```python
from build123d import *

# Parameters (mm, degrees)
SKETCH1_R           = 10
BOSS_EXTRUDE3_DEPTH = 5
SKETCH3_W           = 60
SKETCH3_H           = 50
BOSS_EXTRUDE4_DEPTH = 5
SKETCH9_R           = 12.5
CUT_EXTRUDE3_DEPTH  = 2.5


with BuildPart() as part:
    # Sketch1 → Boss-Extrude3 (new body)
    with BuildSketch(Plane(origin=(0, 0, 0), x_dir=(0, 0, -1), z_dir=(1, 0, 0))):
        with BuildLine():
            Line((0, 0), (50, 0))
            Line((50, 0), (50, -20))
            Line((50, -20), (-18.826787969, -96.735647895))
            ThreePointArc((-18.826787969, -96.735647895), (-38.641397295, -98.984562701), (-43.183296189, -79.566851328))
            Line((-43.183296189, -79.566851328), (0, 0))
        make_face()
        with Locations((-29.998149885, -86.722822296)):
            Circle(SKETCH1_R, mode=Mode.SUBTRACT)
    extrude(amount=BOSS_EXTRUDE3_DEPTH)


with BuildPart() as body_2:
    # Mirror6: mirrored copy
    add(part.part.mirror(Plane(origin=(30, 0, 0), x_dir=(0, 0, 1), z_dir=(1, 0, 0))))


with BuildPart() as part_1:
    add(part.part)

    add(body_2.part)  # Boss-Extrude4 merges body 2
    # Sketch3 → Boss-Extrude4 (add)
    with BuildSketch(Plane(origin=(0, 0, 0), x_dir=(1, 0, 0), z_dir=(0, 1, 0))):
        with Locations((30, 25)):
            Rectangle(SKETCH3_W, SKETCH3_H)
    extrude(amount=BOSS_EXTRUDE4_DEPTH)

    # Sketch9 → Cut-Extrude3 (cut)
    with BuildSketch(Plane(origin=(0, 5, 0), x_dir=(1, 0, 0), z_dir=(0, 1, 0))):
        with Locations((30, 25)):
            Circle(SKETCH9_R)
    extrude(amount=-CUT_EXTRUDE3_DEPTH, mode=Mode.SUBTRACT)


solid = part_1.part
```
Verification items for the finished model (mm, model axes). A direction names the side the tool comes from. Give positions to 0.01 mm unless a question says otherwise; leave off trailing zeros. Write each loop counter-clockwise with the first axis right and the second up, starting at its lowest first coordinate (ties: lowest second). Pieces come first, ordered by that corner, then holes. Notation, with made-up numbers: M -33.75,-38 L -6.75,-38 A33 ccw -6.75,-3 Z; hole C 9.25,59 d6. An arc over 180 degrees is marked long. One line per question, with ' | ' between items.
1) Section check C-C on y = -44.5. Enter the section's corners in (x, z), plus the area to 3 significant figures.
Result:
outline: M 0,-28.03 L 5,-28.03 L 5,24.15 L 0,24.15 Z; M 55,-28.03 L 60,-28.03 L 60,24.15 L 55,24.15 Z | area: 522 mm2
2) Set-up check for faces 1 (the flat face through (0, -37, -2)), 2 (the flat face through (30, 2.5, -25)), 3 (the flat face through (57.54, -57.83, -16.07)), 4 (the flat face through (30, 0, -25)), 5 (the flat face through (30, 2, 0)): record each of +Z, -Z, +X, -X, +Y, -Y from which the full face is reachable in a straight line by a thin tool's end or side.
Result:
face 1: +Z, -Z, -X, +Y, -Y | face 2: +Y | face 3: -Z, +X, -X, -Y | face 4: +Z, -Z, -Y | face 5: +Z, +X, -X, +Y
3) Section check B-B on z = 3. Enter the section's corners in (x, y).
Result:
outline: M 0,-79.09 L 5,-79.09 L 5,-5.53 L 0,-5.53 Z; M 55,-79.09 L 60,-79.09 L 60,-5.53 L 55,-5.53 Z
4) Section check A-A on y = -84. Enter the section's corners in (x, z), plus the area to 3 significant figures.
Result:
outline: M 0,7.4 L 5,7.4 L 5,20.38 L 0,20.38 Z; M 0,39.62 L 5,39.62 L 5,44.75 L 0,44.75 Z; M 55,7.4 L 60,7.4 L 60,20.38 L 55,20.38 Z; M 55,39.62 L 60,39.62 L 60,44.75 L 55,44.75 Z | area: 181 mm2
5) Mould release check, pull along Z, two halves, no side actions. Record for faces 6 (the cylindrical face through (20.08, 3.768, -17.394)), 7 (the cylindrical face through (57.54, -99.16, 38.39)), 8 (the flat face through (57.535, -40.34, 21.894)), 9 (the flat face through (23, 5, -36)): released by +Z, released by -Z, zero draft, split by the parting line, or undercut.
Result:
face 6: undercut | face 7: split by the parting line | face 8: released by +Z | face 9: zero draft
6) Section check D-D on z = 30. Enter the section's corners in (x, y).
Result:
outline: M 0,-101.72 L 5,-101.72 L 5,-96.72 L 0,-96.72 Z; M 0,-76.72 L 5,-76.72 L 5,-55.28 L 0,-55.28 Z; M 55,-101.72 L 60,-101.72 L 60,-96.72 L 55,-96.72 Z; M 55,-76.72 L 60,-76.72 L 60,-55.28 L 55,-55.28 Z
7) Thickness scan on line 1 along Z through (x, y) = (30, 3.6); line 2 along X through (y, z) = (-21.5, 7); line 3 along X through (y, z) = (3.5, -25). Record the ranges inside material, lowest first. Write a range as [from, to].
Result:
line 1: z = [-50, -37.5], [-12.5, 0] | line 2: x = [0, 5], [55, 60] | line 3: x = [0, 17.5], [42.5, 60]
8) Gauge pin test, flat ends, axial feed: pin 1 Ø7.5 at (x, z) = (27, -27.5) entering from +Y; pin 2 Ø4 at (x, y) = (34, 2) entering from +Z. Record the tip position at first contact, or that the pin passes through.
Result:
pin 1: stops at y = 2.5 | pin 2: stops at z = 0
